```python
from build123d import *

# Parameters (mm, degrees)
SKETCH1_W                       = 132
SKETCH1_H                       = 36
BOSS_EXTRUDE1_DEPTH             = 5
SKETCH2_W                       = 26
SKETCH2_H                       = 5
CUT_EXTRUDE1_DEPTH              = 67
CUT_EXTRUDE1_DEPTH_BACK         = 67
CHAMFER1_SIZE                   = 1
TAP_DRILL_FOR_M4X0_7_TAP1_D     = 3.3
TAP_DRILL_FOR_M4X0_7_TAP1_DEPTH = 14
TAP_DRILL_FOR_M4X0_7_TAP1_TIP   = 0.991420021


with BuildPart() as part:
    # Sketch1 → Boss-Extrude1 (new body, symmetric)
    with BuildSketch(Plane(origin=(0, 0, 0), x_dir=(1, 0, 0), z_dir=(0, 1, 0))):
        Rectangle(SKETCH1_W, SKETCH1_H)
    extrude(amount=BOSS_EXTRUDE1_DEPTH, both=True)

    # Sketch2 → Cut-Extrude1 (cut, two sides)
    with BuildSketch(Plane(origin=(0, 0, 0), x_dir=(0, 0, -1), z_dir=(1, 0, 0))) as cut_extrude1_sk:
        with Locations((0, -2.5)):
            Rectangle(SKETCH2_W, SKETCH2_H)
    extrude(amount=CUT_EXTRUDE1_DEPTH, mode=Mode.SUBTRACT)
    extrude(cut_extrude1_sk.sketch, amount=-CUT_EXTRUDE1_DEPTH_BACK, mode=Mode.SUBTRACT)

    # Chamfer1
    chamfer1_edges = [part.edges().sort_by_distance(p)[0] for p in [
        (-66, -2.5, 13),
        (-66, -5, -15.5),
        (-66, 0, 0),
        (-66, -2.5, -13),
        (0, -5, 13),
        (66, -5, -15.5),
        (66, -2.5, -13),
        (66, 0, 0),
        (66, -2.5, 13),
        (0, -5, 18),
        (66, 0, 18),
        (66, 5, 0),
        (0, 5, -18),
        (-66, 5, 0),
        (0, 5, 18),
        (-66, 0, 18),
        (0, -5, -13),
    ]]
    chamfer(chamfer1_edges, length=CHAMFER1_SIZE)

    # Tap Drill for M4x0.7 Tap1
    with Locations(Plane(origin=(-96, 5, 18), x_dir=(1, 0, 0), z_dir=(0, 1, 0))):
        with Locations((55, 27), (122, 27), (55, 9), (122, 9)):
            Hole(TAP_DRILL_FOR_M4X0_7_TAP1_D / 2, depth=TAP_DRILL_FOR_M4X0_7_TAP1_DEPTH)
            with Locations((0, 0, -(TAP_DRILL_FOR_M4X0_7_TAP1_DEPTH + TAP_DRILL_FOR_M4X0_7_TAP1_TIP / 2))):  # 118° drill point
                Cone(0, TAP_DRILL_FOR_M4X0_7_TAP1_D / 2, TAP_DRILL_FOR_M4X0_7_TAP1_TIP, mode=Mode.SUBTRACT)


solid = part.part
```
Input: part model. Units: mm. Frame: model coordinates. A direction names the side the tool comes from. Round coordinates to 2 decimals unless told otherwise and drop trailing zeros. Loops run counter-clockwise (first coordinate to the right, second up) from the corner with the lowest first, then second, coordinate; pieces in that order, holes last. Notation, with made-up numbers: (-6.5, -7) -> (22.5, -7) arc R20 cw to (22.5, 2) -> close; hole circle Ø11 at (72, 75.5). An arc over 180 degrees is marked (long way). Write each question's results on one line, items separated by ' | '.
1. Section C-C (x = -37). Return loops of the section in (y, z), and give its area (4 significant figures).
Geometry results:
outline: (-5, -18) -> (4, -18) -> (5, -17) -> (5, 17) -> (4, 18) -> (-4, 18) -> (-5, 17) -> (-5, 14) -> (-4, 13) -> (0, 13) -> (0, -13) -> (-4, -13) -> (-5, -14) -> close | area: 227.5 mm2
2. First-contact query: P1, Ø4, axis at x = -41, z = 9, coming from the -Y side; P2, Ø1.5, axis at x = -0.5, z = 13, coming from the -Y side; P3, Ø2.5, axis at x = 26, z = -9, coming from the -Y side; P4, Ø4, axis at y = -2, z = 13, coming from the +X side. Flat tips, straight axial feed; report the tip coordinate or a pass-through.
Geometry results:
P1: y = 0 | P2: y = -4.75 | P3: through | P4: x = 66
3. Section B-B (x = 26). Return loops of the section in (y, z).
Geometry results:
outline: (-5, -18) -> (4, -18) -> (5, -17) -> (5, -10.65) -> (0, -10.65) -> (0, -13) -> (-4, -13) -> (-5, -14) -> close; (-5, 14) -> (-4, 13) -> (0, 13) -> (0, 10.65) -> (5, 10.65) -> (5, 17) -> (4, 18) -> (-4, 18) -> (-5, 17) -> close; (0, -7.35) -> (5, -7.35) -> (5, 7.35) -> (0, 7.35) -> close
4. Set-up query: faces 1 (the face through (1, -2, -13)), 2 (the face through (27.31, 2.46, -8)). Return all of +Z, -Z, +X, -X, +Y, -Y with unobstructed straight access to the full face (end or side cutting, diameter ignored); none if empty.
Geometry results:
face 1: +X, -X, -Y | face 2: +Y, -Y
5. Section D-D (z = -2). Return loops of the section in (x, y), and give its area (3 significant figures).
Geometry results:
outline: (-66, 1) -> (-65, 0) -> (65, 0) -> (66, 1) -> (66, 4) -> (65, 5) -> (-65, 5) -> (-66, 4) -> close | area: 658 mm2
6. Section A-A (z = 9). Return loops of the section in (x, y).
Geometry results:
outline: (-66, 1) -> (-65, 0) -> (-42.65, 0) -> (-42.65, 5) -> (-65, 5) -> (-66, 4) -> close; (-39.35, 0) -> (24.35, 0) -> (24.35, 5) -> (-39.35, 5) -> close; (27.65, 0) -> (65, 0) -> (66, 1) -> (66, 4) -> (65, 5) -> (27.65, 5) -> close
7. Ray query, line 1 (Z direction, x = 26, y = 1.8); line 2 (X direction, y = 3.45, z = 9); line 3 (Z direction, x = 21, y = -2.5). Return the intervals inside material, ascending. Write a range as from..to.
Geometry results:
line 1: -18..-10.65, -7.35..7.35, 10.65..18 | line 2: -66..-42.65, -39.35..24.35, 27.65..66 | line 3: -18..-13, 13..18
8. Mould query, pull axis Z, two halves, no side actions, for faces 3 (the face through (-39.35, 2.46, -9.07)), 4 (the face through (-1, 5, 0)), 5 (the face through (-1, 0, 18)), 6 (the face through (-1, 0, -18)). Classes: +Z half, -Z half, draft (parallel to the pull), parting line (faces both ways), or undercut.
Geometry results:
face 3: undercut | face 4: draft | face 5: +Z half | face 6: -Z half
